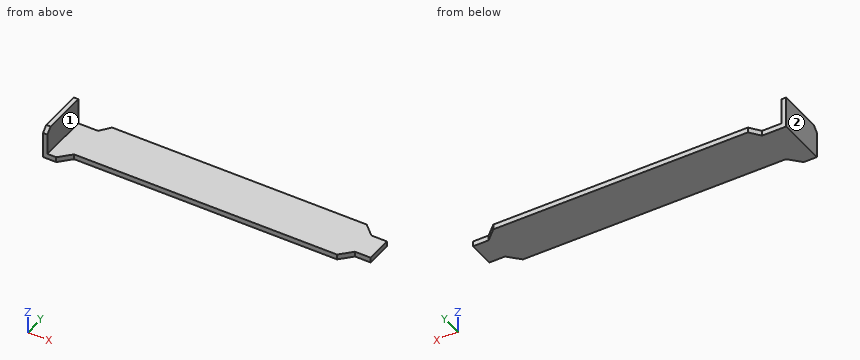
```python
from build123d import *

# Parameters (mm, degrees)
F0_W     = 1.681574
F0_H     = 19.19315
F1_DEPTH = 12
F2_DEPTH = 2
F3_SIZE  = 2


with BuildPart() as f1:
    # F0 (on Top) → F1 (new body)
    with BuildSketch(Plane.XY):
        with Locations((-54.7731, -4.393613)):
            Rectangle(F0_W, F0_H)
    extrude(amount=F1_DEPTH)

    # F0 (on Top) → F2 (join)
    with BuildSketch(Plane.XY):
        Polygon((54.688916, 9.13409), (-43.35802, 9.13409), (-46.364177, 5.202962), (-53.932313, 5.202962), (-53.932313, -13.990188), (-50.526548, -13.990188), (-46.364177, -9.596575), (54.920163, -9.596575), (59.082527, -5.202962), (65.094844, -5.202962), (65.094844, 4.97172), (59.082527, 4.97172), align=None)
        with Locations((-54.7731, -4.393613)):
            Rectangle(F0_W, F0_H)
    extrude(amount=F2_DEPTH)

    # F3
    f3_edges = [f1.edges().sort_by_distance(p)[0] for p in [
        (-54.7731, -13.990188, 12),
    ]]
    chamfer(f3_edges, length=F3_SIZE)


solid = f1.part
```
CAD build for the part. Positions are in the model's coordinates, mm. Face numbers are marked on the shaded views. A direction names the side the tool comes from. Round coordinates to 2 decimals unless told otherwise and drop trailing zeros. Write each loop counter-clockwise with the first axis right and the second up, starting at its lowest first coordinate (ties: lowest second). Pieces come first, ordered by that corner, then holes. Notation, with made-up numbers: (-8, 44) - (-3, 44) arc R7 cw to (-3, 57) - close; hole circle Ø1 at (42, -17.5). An arc over 180 degrees is marked (long way). Return JSON: item names as keys, results as strings. Group by question number.
Item 1: Band-saw the part on C-C on x = 33. List the corners of the cut face in (y, z).
Item 2: Probe probe 1 along Z at (x, y) = (-34, 7); probe 2 along Y at (x, z) = (37, 1.5); probe 3 along X at (y, z) = (-2.5, 7). List the from-to ranges inside material, lowest first.
Item 3: Band-saw the part on B-B on y = 1. List the corners of the cut face in (x, z), plus the area to 3 significant figures.
Item 4: 3-axis set-ups, long thin cutter, end or side, ignore diameter. For the marked faces 1 and 2: which of +Z, -Z, +X, -X, +Y, -Y reach the whole face in a straight line?
Item 5: Flat gauge pins, fed straight in: pin 1 Ø1 at (y, z) = (-8, 9) entering from +X; pin 2 Ø2 at (x, y) = (51.5, -2.5) entering from +Z; pin 3 Ø1 at (x, z) = (62.5, 1) entering from -Y. Where does each tip first touch, or does it go through?
Item 6: Band-saw the part on A-A on z = 1. List the corners of the cut face in (x, y), plus the area to 3 significant figures.
Resolved:
{
 "1": {"outline": "(-9.6, 0) - (9.13, 0) - (9.13, 2) - (-9.6, 2) - close"},
 "2": {"probe 1": "z = 0 to 2", "probe 2": "y = -9.6 to 9.13", "probe 3": "x = -55.61 to -53.93"},
 "3": {"outline": "(-55.61, 0) - (65.09, 0) - (65.09, 2) - (-53.93, 2) - (-53.93, 12) - (-55.61, 12) - close", "area": "258 mm²"},
 "4": {"face 1": "+Z, +X, +Y, -Y", "face 2": "+Z, -Z, -X, +Y, -Y"},
 "5": {"pin 1": "stops at x = -53.93", "pin 2": "stops at z = 2", "pin 3": "stops at y = -5.2"},
 "6": {"outline": "(-55.61, -13.99) - (-50.53, -13.99) - (-46.36, -9.6) - (54.92, -9.6) - (59.08, -5.2) - (65.09, -5.2) - (65.09, 4.97) - (59.08, 4.97) - (54.69, 9.13) - (-43.36, 9.13) - (-46.36, 5.2) - (-55.61, 5.2) - close", "area": "2,180 mm²"}
}
